The model under review builds one solid part; all positions refer to its coordinate system, in mm. Face numbers are marked on the shaded views. A direction names the side the tool comes from. Round coordinates to 2 decimals unless told otherwise and drop trailing zeros. Order: outer loops, then holes, each group sorted by start corner. A loop starts at its lowest first (then second) coordinate and runs counter-clockwise, first axis right, second up. Notation, with made-up numbers: (-13.5, -23) - (27.5, -23) arc R20 cw to (27.5, 3) - close; hole circle Ø4 at (75, -3). An arc over 180 degrees is marked (long way). One line per question, with ' | ' between items. Start each with the question number.
Item 1: Add section A-A on z = -26. State the section outline as (x, y) points.
Item 2: For L1, parallel to Y at x = 45, z = -18.5; L2, parallel to X at y = 20, z = -37; L3, parallel to X at y = 10.75, z = -8.5, list the stretches that pass through material, from the lowest coordinate up. Write a range as [from, to].
Item 3: Tool access review of the marked faces 1 and 2: name each direction out of +Z, -Z, +X, -X, +Y, -Y from which nothing blocks a thin tool from reaching the whole face with its end or side.
Item 4: Insertion check: pin 1 Ø20 at (x, z) = (27.5, -13.5) entering from +Y; pin 2 Ø6.5 at (x, z) = (6, -27.5) entering from -Y; pin 3 Ø4 at (y, z) = (-2.5, -25) entering from +X. Each pin has a flat end and moves straight along its axis. Give the tip position at first contact, or say it passes through.
Item 5: Add section B-B on y = 5.75. State the section outline as (x, z) points.
Item 6: Add section C-C on x = 20.5. State the section outline as (y, z) points.
Item 7: Draft analysis for pull direction X (two halves, no side actions). For the marked faces 3, 4, 5 and 6, state which applies: +X half, -X half, draft (parallel to the pull), parting line (faces both ways), or undercut.
Item 8: Add section D-D on z = -21.5. State the section outline as (x, y) points, and give its area (3 significant figures).
from build123d import *

# Parameters (mm, degrees)
SKETCH1_W                = 50
SKETCH1_H                = 40
BOSS_EXTRUDE2_DEPTH      = 5
SKETCH2_W                = 2
SKETCH2_H                = 40
BOSS_EXTRUDE4_DEPTH      = 12
SKETCH3_W                = 10
SKETCH3_H                = 40
BOSS_EXTRUDE5_DEPTH      = 5
BOSS_EXTRUDE6_DEPTH      = 15
BOSS_EXTRUDE6_DEPTH_BACK = 15
SKETCH5_R                = 1.5


with BuildPart() as part:
    # Sketch1 → Boss-Extrude2 (new body)
    with BuildSketch(Plane(origin=(0, 0, 0), x_dir=(1, 0, 0), z_dir=(0, 1, 0))):
        with Locations((25, 20)):
            Rectangle(SKETCH1_W, SKETCH1_H)
    extrude(amount=BOSS_EXTRUDE2_DEPTH)

    # Sketch2 → Boss-Extrude4 (add)
    with BuildSketch(Plane(origin=(0, 5, 0), x_dir=(1, 0, 0), z_dir=(0, 1, 0))):
        with Locations((1, 20)):
            Rectangle(SKETCH2_W, SKETCH2_H)
        with Locations((49, 20)):
            Rectangle(SKETCH2_W, SKETCH2_H)
    extrude(amount=BOSS_EXTRUDE4_DEPTH)

    # Sketch3 → Boss-Extrude5 (add)
    with BuildSketch(Plane(origin=(0, 17, 0), x_dir=(1, 0, 0), z_dir=(0, 1, 0))):
        with Locations((5, 20)):
            Rectangle(SKETCH3_W, SKETCH3_H)
        with Locations((45, 20)):
            Rectangle(SKETCH3_W, SKETCH3_H)
    extrude(amount=BOSS_EXTRUDE5_DEPTH)

    # Sketch5 → Boss-Extrude6 (add, two sides: drawn at the far end of the back side and taken through both)
    with BuildSketch(Plane(origin=(25, 0, 0), x_dir=(0, 0, -1), z_dir=(1, 0, 0)).offset(-BOSS_EXTRUDE6_DEPTH_BACK)):
        with BuildLine():
            Line((23.5, 0), (23.5, -2.5))
            ThreePointArc((23.5, -2.5), (26, -5), (28.5, -2.5))
            Line((28.5, -2.5), (28.5, 0))
            Line((28.5, 0), (23.5, 0))
        make_face()
        with Locations((26, -2)):
            Circle(SKETCH5_R, mode=Mode.SUBTRACT)
    extrude(amount=BOSS_EXTRUDE6_DEPTH + BOSS_EXTRUDE6_DEPTH_BACK)


solid = part.part
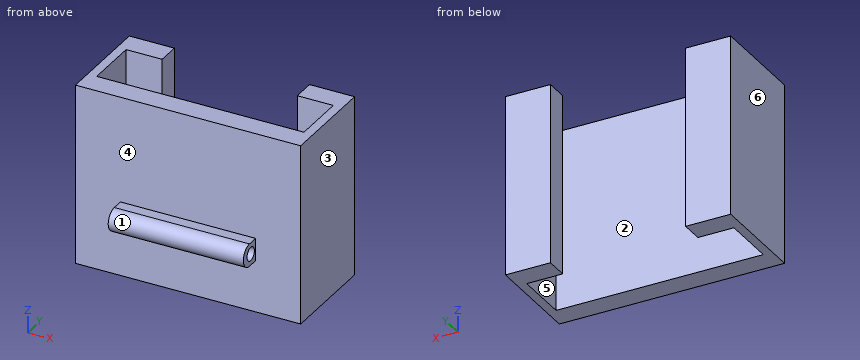
Determined:
1) outline: (0, 0) - (10, 0) - (10, -0.5) - (40, -0.5) - (40, 0) - (50, 0) - (50, 22) - (40, 22) - (40, 17) - (48, 17) - (48, 5) - (2, 5) - (2, 17) - (10, 17) - (10, 22) - (0, 22) - close; (10, -5) - (40, -5) - (40, -3.5) - (10, -3.5) - close
2) L1: [0, 5], [17, 22] | L2: [0, 10], [40, 50] | L3: [0, 2], [48, 50]
3) face 1: +X, -X, -Y | face 2: +Z, -Z
4) pin 1: y = 5 | pin 2: y = 0 | pin 3: x = 40
5) outline: (0, -40) - (2, -40) - (2, 0) - (0, 0) - close; (48, -40) - (50, -40) - (50, 0) - (48, 0) - close
6) outline: (-2.5, -28.5) - (0, -28.5) - (0, -40) - (5, -40) - (5, 0) - (0, 0) - (0, -23.5) - (-2.5, -23.5) arc R2.5 ccw to start; hole circle Ø3 at (-2, -26)
7) face 3: +X half | face 4: draft | face 5: undercut | face 6: -X half
8) outline: (0, 0) - (50, 0) - (50, 22) - (40, 22) - (40, 17) - (48, 17) - (48, 5) - (2, 5) - (2, 17) - (10, 17) - (10, 22) - (0, 22) - close | area: 398 mm2
